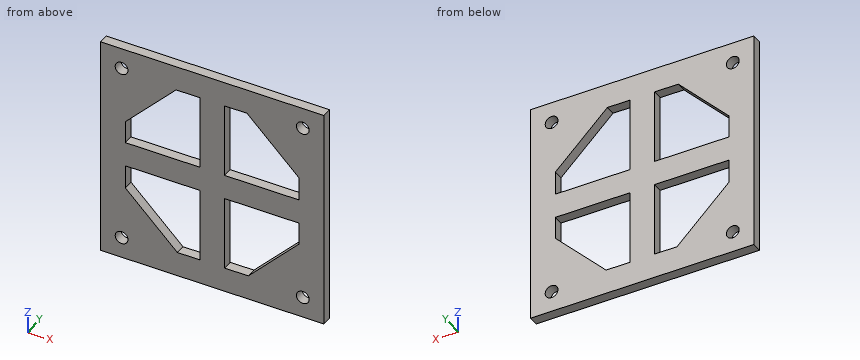
```python
from build123d import *

# Parameters (mm, degrees)
SKETCH2_W           = 45
SKETCH2_H           = 45
BOSS_EXTRUDE1_DEPTH = 2
CUT_EXTRUDE1_DEPTH  = 2
SKETCH7_R           = 1.289214756
CUT_EXTRUDE2_DEPTH  = 2
CIRPATTERN1_COUNT   = 4


with BuildPart() as part:
    # Sketch2 → Boss-Extrude1 (new body)
    with BuildSketch(Plane(origin=(0, 0, 0), x_dir=(1, 0, 0), z_dir=(0, 1, 0))):
        Rectangle(SKETCH2_W, SKETCH2_H)
    extrude(amount=BOSS_EXTRUDE1_DEPTH)

    # Sketch4 → Cut-Extrude1 (cut)
    with BuildSketch(Plane.XZ):
        Polygon((7.021849723, 17.5), (17.5, 7.271715562), (17.5, 2.5), (2.5, 2.5), (2.5, 17.5), align=None)
    cut_extrude1 = extrude(amount=-CUT_EXTRUDE1_DEPTH, mode=Mode.SUBTRACT)

    # Sketch7 → Cut-Extrude2 (cut)
    with BuildSketch(Plane.XZ):
        with Locations((18.257359313, 18.257359313)):
            Circle(SKETCH7_R)
    cut_extrude2 = extrude(amount=-CUT_EXTRUDE2_DEPTH, mode=Mode.SUBTRACT)

    # CirPattern1: Cut-Extrude1, Cut-Extrude2 ×4 about axis
    cirpattern1_axis = Axis((0, 0, 0), (0, 1, 0))
    for i in range(1, CIRPATTERN1_COUNT):
        add(cut_extrude1.rotate(cirpattern1_axis, i * 360 / CIRPATTERN1_COUNT), mode=Mode.SUBTRACT)
        add(cut_extrude2.rotate(cirpattern1_axis, i * 360 / CIRPATTERN1_COUNT), mode=Mode.SUBTRACT)


solid = part.part
```
CAD build for the part. Positions are in the model's coordinates, mm. Round coordinates to 2 decimals unless told otherwise and drop trailing zeros. Write each loop counter-clockwise with the first axis right and the second up, starting at its lowest first coordinate (ties: lowest second). Pieces come first, ordered by that corner, then holes. Notation, with made-up numbers: (3.5, 59) -> (22.5, 59) arc R27 ccw to (22.5, 83) -> close; hole circle Ø6 at (-10.5, 7). An arc over 180 degrees is marked (long way). Answer in a Markdown table with one row per item. Add a question column.
Item 1: Saw through at C-C, the plane y = 0.5. Count the separate pieces of the cut face and the enclosed holes in it, then the cut area to 3 significant figures.
Item 2: Saw through at B-B, the plane z = -19. Write the cut outline in (x, y).
Item 3: Drop a flat-ended pin along its axis: pin 1 Ø3 at (x, z) = (-18.26, 18.26) entering from +Y. Give the stop position or say it passes through.
Item 4: Drill centre lines: line 1 (X direction, y = 1.25, z = 4); line 2 (X direction, y = 0.6, z = 18). Where is each one in solid material? Low to high. Write a range as from..to.
Item 5: Saw through at A-A, the plane x = 12. Write the cut outline in (y, z), then the cut area to 3 significant figures.
Findings below:
| question | item | result |
|---|---|---|
| 1 | separate pieces | 1 |
| 1 | enclosed holes | 8 |
| 1 | area | 1,320 mm^2 |
| 2 | outline | (-22.5, 0) -> (-19.31, 0) -> (-19.31, 2) -> (-22.5, 2) -> close; (-17.2, 0) -> (17.2, 0) -> (17.2, 2) -> (-17.2, 2) -> close; (19.31, 0) -> (22.5, 0) -> (22.5, 2) -> (19.31, 2) -> close |
| 3 | pin 1 | stops at y = 2 |
| 4 | line 1 | x = -22.5..-17.5, -2.5..2.5, 17.5..22.5 |
| 4 | line 2 | x = -22.5..-19.52, -16.99..16.99, 19.52..22.5 |
| 5 | outline | (0, -22.5) -> (2, -22.5) -> (2, -12.66) -> (0, -12.66) -> close; (0, -2.5) -> (2, -2.5) -> (2, 2.5) -> (0, 2.5) -> close; (0, 12.64) -> (2, 12.64) -> (2, 22.5) -> (0, 22.5) -> close |
| 5 | area | 49.4 mm^2 |
